CAD build for the part. Positions are in the model's coordinates, mm. Face numbers are marked on the shaded views. A direction names the side the tool comes from. Coordinates: 2 decimals unless noted, no trailing zeros. Write each loop counter-clockwise with the first axis right and the second up, starting at its lowest first coordinate (ties: lowest second). Pieces come first, ordered by that corner, then holes. Notation, with made-up numbers: (11.25, 19) - (22.25, 19) arc R16 ccw to (22.25, 35) - close; hole circle Ø3 at (15.5, 29). An arc over 180 degrees is marked (long way). Answer in a Markdown table with one row per item. Add a question column.
Q1. Band-saw the part on D-D (x = -36). List the corners of the cut face in (y, z), and give its area (3 significant figures).
Q2. Pin check, flat tips, straight feed: pin 1 (8 mm diameter, centred on x = -35, y = -5.5, fed in from +Z); pin 2 (5 mm diameter, centred on y = 31.25, z = 5, fed in from +X); pin 3 (3.5 mm diameter, centred on x = -42.5, z = 4, fed in from +Y); pin 4 (3 mm diameter, centred on y = 28.5, z = 3, fed in from -X). Stop position of each tip, or through.
Q3. Band-saw the part on B-B (y = 29.5). List the corners of the cut face in (x, z), and give its area (3 significant figures).
Q4. Band-saw the part on C-C (x = 27). List the corners of the cut face in (y, z).
Q5. 3-axis set-ups, long thin cutter, end or side, ignore diameter. For the marked faces 1, 2, 3, 4 and 5: which of +Z, -Z, +X, -X, +Y, -Y reach the whole face in a straight line?
Q6. Drill centre lines: line 1 along Z through (x, y) = (-15, 31.25); line 2 along X through (y, z) = (28.5, 8); line 3 along Y through (x, z) = (2.5, 1.5). Where is each one in solid material? Low to high. Write a range as from..to.
Q7. Band-saw the part on A-A (z = 5). List the corners of the cut face in (x, y), and give its area (3 significant figures).
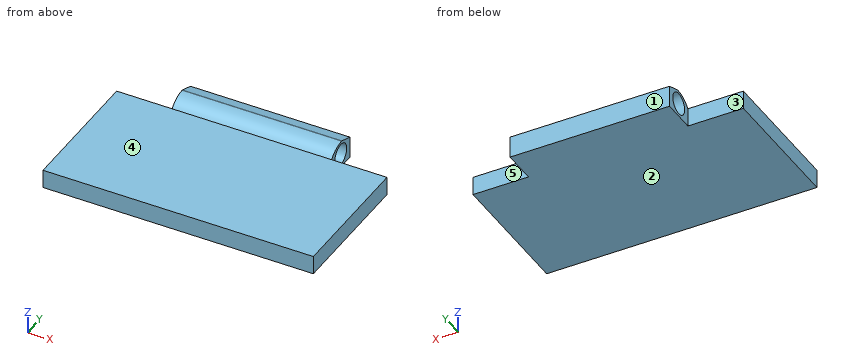
```python
from build123d import *

# Parameters (mm, degrees)
F0_W        = 59
F0_H        = 12.5
F1_DEPTH    = 10
F2_DEPTH    = 6.9
F3_R        = 4
F4_DEPTH    = 59
F5_T1_DEPTH = 92.9816126751
F6_SIZE2    = 5.4949548389
F6_SIZE     = 2


# Not quite as in the source:
# - a fillet or chamfer that OpenCascade refuses, or shapes differently, is made with other operations: its cross-section is extruded or revolved along the edge and cut away or added


with BuildPart() as f1:
    # F0 (on Top) → F1 (new body)
    with BuildSketch(Plane.XY):
        with Locations((0, 31.25)):
            Rectangle(F0_W, F0_H)
    extrude(amount=F1_DEPTH)

    # F0 (on Top) → F2 (join)
    with BuildSketch(Plane.XY):
        Polygon((-50, -25), (50, -25), (50, 25), (29.5, 25), (-29.5, 25), (-50, 25), align=None)
    extrude(amount=F2_DEPTH)

    # F3 (on face) → F4 (cut, through all)
    with BuildSketch(Plane.YZ.offset(29.5)):
        with Locations((31.25, 5)):
            Circle(F3_R)
    extrude(amount=-F4_DEPTH, mode=Mode.SUBTRACT)

    # F5: fillet of radius 9 on 1 edges, made by hand

    # F5_s2 → F5_t1 (cut)
    with BuildSketch(Plane.YZ.offset(-46.4908063375)):
        with BuildLine():
            ThreePointArc((25, 6.9), (28.0613526556, 9.1884064384), (31.796322535, 10))
            Line((31.796322535, 10), (25, 10))
            Line((25, 10), (25, 6.9))
        make_face()
    extrude(amount=F5_T1_DEPTH, mode=Mode.SUBTRACT)

    # F6
    f6_edges = [f1.edges().sort_by_distance(p)[0] for p in [
        (0, 37.5, 10),
    ]]
    f6_side = f1.faces().sort_by_distance((0, 37.5, 5))[0]
    chamfer(f6_edges, length=F6_SIZE, length2=F6_SIZE2, reference=f6_side)


solid = f1.part
```
Checked values:
| question | item | result |
|---|---|---|
| 1 | outline | (-25, 0) - (25, 0) - (25, 6.9) - (-25, 6.9) - close |
| 1 | area | 345 mm² |
| 2 | pin 1 | stops at z = 6.9 |
| 2 | pin 2 | passes through |
| 2 | pin 3 | stops at y = 25 |
| 2 | pin 4 | stops at x = -29.5 |
| 3 | outline | (-29.5, 0) - (29.5, 0) - (29.5, 1.4) - (-29.5, 1.4) - close; (-29.5, 8.6) - (29.5, 8.6) - (29.5, 9.7) - (-29.5, 9.7) - close |
| 3 | area | 148 mm² |
| 4 | outline | (-25, 0) - (37.5, 0) - (37.5, 8) - (32.01, 10) - (31.8, 10) arc R9 ccw to (25, 6.9) - (-25, 6.9) - close; hole circle Ø8 at (31.25, 5) |
| 5 | face 1 | +Z, -Z, +X, -X, +Y |
| 5 | face 2 | -Z, +X, -X, +Y, -Y |
| 5 | face 3 | +Z, -Z, -X, +Y |
| 5 | face 4 | +Z, +X, -X, -Y |
| 5 | face 5 | +Z, -Z, +X, +Y |
| 6 | line 1 | z = 0..1, 9..9.98 |
| 6 | line 2 | x = -29.5..29.5 |
| 6 | line 3 | y = -25..29.31, 33.19..37.5 |
| 7 | outline | (-50, -25) - (50, -25) - (50, 25) - (29.5, 25) - (29.5, 27.25) - (-29.5, 27.25) - (-29.5, 25) - (-50, 25) - close; (-29.5, 35.25) - (29.5, 35.25) - (29.5, 37.5) - (-29.5, 37.5) - close |
| 7 | area | 5,270 mm² |
